Geometry: final body of the model. Coordinates: model frame, mm. A direction names the side the tool comes from. Round coordinates to 2 decimals unless told otherwise and drop trailing zeros. Loops run counter-clockwise (first coordinate to the right, second up) from the corner with the lowest first, then second, coordinate; pieces in that order, holes last. Notation, with made-up numbers: (63, -12.5) -> (75, -12.5) arc R14 cw to (75, -7.5) -> close; hole circle Ø3 at (65, 21.25). An arc over 180 degrees is marked (long way). Answer in a Markdown table with one row per item.
```python
from build123d import *

# Parameters (mm, degrees)
SKETCH1_R           = 20
SKETCH1_R_2         = 10
BOSS_EXTRUDE1_DEPTH = 3
SKETCH2_W           = 40
SKETCH2_H           = 3
BOSS_EXTRUDE2_DEPTH = 42.8
FILLET1_R           = 0.5
FILLET2_R           = 3.5
FILLET3_R           = 4
SKETCH3_R           = 1.75
CUT_EXTRUDE1_DEPTH  = 10


with BuildPart() as part:
    # Sketch1 → Boss-Extrude1 (new body)
    with BuildSketch(Plane(origin=(0, 0, 0), x_dir=(0, 0, -1), z_dir=(1, 0, 0))):
        with BuildLine():
            Line((-20, 27.2), (-20, 0))
            ThreePointArc((-20, 0), (0, 20), (20, 0))
            Line((20, 0), (20, 27.2))
            Line((20, 27.2), (-20, 27.2))
        make_face()
        Circle(SKETCH1_R)
        Circle(SKETCH1_R_2, mode=Mode.SUBTRACT)
    extrude(amount=BOSS_EXTRUDE1_DEPTH)

    # Sketch2 → Boss-Extrude2 (add)
    with BuildSketch(Plane(origin=(3, 0, 0), x_dir=(0, 0, -1), z_dir=(1, 0, 0))):
        with Locations((0, 25.7)):
            Rectangle(SKETCH2_W, SKETCH2_H)
    extrude(amount=-BOSS_EXTRUDE2_DEPTH)

    # Fillet1
    fillet1_edges = [part.edges().sort_by_distance(p)[0] for p in [
        (0, 24.2, 0),
    ]]
    fillet(fillet1_edges, radius=FILLET1_R)

    # Fillet2
    fillet2_edges = [part.edges().sort_by_distance(p)[0] for p in [
        (3, 27.2, 0),
    ]]
    fillet(fillet2_edges, radius=FILLET2_R)

    # Fillet3
    fillet3_edges = [part.edges().sort_by_distance(p)[0] for p in [
        (-39.8, 25.7, 20),
        (-39.8, 25.7, -20),
    ]]
    fillet(fillet3_edges, radius=FILLET3_R)

    # Sketch3 → Cut-Extrude1 (cut)
    with BuildSketch(Plane(origin=(0, 27.2, 0), x_dir=(1, 0, 0), z_dir=(0, 1, 0))):
        with Locations((-29.55, 15.05)):
            Circle(SKETCH3_R)
        with Locations((-5.45, 15.05)):
            Circle(SKETCH3_R)
        with Locations((-29.55, -15.05)):
            Circle(SKETCH3_R)
        with Locations((-5.45, -15.05)):
            Circle(SKETCH3_R)
    extrude(amount=-CUT_EXTRUDE1_DEPTH, mode=Mode.SUBTRACT)


solid = part.part
```
Item 1: Section query A-A, the plane x = -29.55. Output: boundary loops of the cut face in (y, z), and give its area (3 significant figures).
Ans:
| item | result |
|---|---|
| outline | (24.2, -20) -> (27.2, -20) -> (27.2, -16.8) -> (24.2, -16.8) -> close; (24.2, -13.3) -> (27.2, -13.3) -> (27.2, 13.3) -> (24.2, 13.3) -> close; (24.2, 16.8) -> (27.2, 16.8) -> (27.2, 20) -> (24.2, 20) -> close |
| area | 99.0 mm2 |
Item 2: Ray query, L1, parallel to Z at x = -29.55, y = 25.6; L2, parallel to Y at x = -1.5, z = -1; L3, parallel to X at y = 25, z = -14. Return the intervals inside material, ascending.
Ans:
| item | result |
|---|---|
| L1 | -20 to -16.8, -13.3 to 13.3, 16.8 to 20 |
| L2 | 24.2 to 27.2 |
| L3 | -39.8 to -30.95, -28.15 to -6.85, -4.05 to 2.75 |
Item 3: Set-up query: faces 4 (the cylindrical face through (2, 26.15, 0.28)), 5 (the flat face through (-20, 24.2, 0)). Return all of +Z, -Z, +X, -X, +Y, -Y with unobstructed straight access to the full face (end or side cutting, diameter ignored); none if empty.
Ans:
| item | result |
|---|---|
| face 4 | +Z, -Z, +X, +Y |
| face 5 | +Z, -Z, -X, -Y |
Item 4: Mould query, pull axis Z, two halves, no side actions, for faces 1 (the cylindrical face through (-6.74, 25.72, -16.23)), 2 (the flat face through (-20, 27.2, 0)), 3 (the cylindrical face through (1, -20, 0)). Classes: released by +Z, released by -Z, zero draft, split by the parting line, or undercut.
Ans:
| item | result |
|---|---|
| face 1 | undercut |
| face 2 | zero draft |
| face 3 | split by the parting line |
Item 5: Section query C-C, the plane z = -6.5. Output: boundary loops of the cut face in (x, y).
Ans:
| item | result |
|---|---|
| outline | (-39.8, 24.2) -> (-0.5, 24.2) arc R0.5 cw to (0, 23.7) -> (0, 7.6) -> (3, 7.6) -> (3, 23.7) arc R3.5 ccw to (-0.5, 27.2) -> (-39.8, 27.2) -> close; (0, -18.91) -> (3, -18.91) -> (3, -7.6) -> (0, -7.6) -> close |
Item 6: Section query D-D, the plane z = -15.05. Output: boundary loops of the cut face in (x, y).
Ans:
| item | result |
|---|---|
| outline | (-39.8, 24.2) -> (-31.3, 24.2) -> (-31.3, 27.2) -> (-39.8, 27.2) -> close; (-27.8, 24.2) -> (-7.2, 24.2) -> (-7.2, 27.2) -> (-27.8, 27.2) -> close; (-3.7, 24.2) -> (-0.5, 24.2) arc R0.5 cw to (0, 23.7) -> (0, -13.17) -> (3, -13.17) -> (3, 23.7) arc R3.5 ccw to (-0.5, 27.2) -> (-3.7, 27.2) -> close |
Item 7: Section query B-B, the plane y = -3.5. Output: boundary loops of the cut face in (x, z).
Ans:
| item | result |
|---|---|
| outline | (0, -19.69) -> (3, -19.69) -> (3, -9.37) -> (0, -9.37) -> close; (0, 9.37) -> (3, 9.37) -> (3, 19.69) -> (0, 19.69) -> close |
Item 8: First-contact query: P1, Ø12, axis at x = -11.5, z = 2.5, coming from the -Y side; P2, Ø2, axis at y = 9.5, z = -15.5, coming from the -X side. Flat tips, straight axial feed; report the tip coordinate or a pass-through.
Ans:
| item | result |
|---|---|
| P1 | y = 24.2 |
| P2 | x = 0 |
